Autodesk Inventor part; units mm, degrees
ref_plane "YZ Plane" through (0, 0, 0) normal (1, 0, 0) x (0, 1, 0)
ref_plane "XZ Plane" through (0, 0, 0) normal (0, 1, 0) x (-1, 0, 0)
ref_plane "XY Plane" through (0, 0, 0) normal (0, 0, 1) x (1, 0, 0)
sketch "Sketch1" plane through (0, 0, 0) normal (0, 0, 1) x (1, 0, 0)
  line L0 (0, 0) -> (236.5375, 0)
  line L1 (527.05, 0) -> (527.05, 248.2464)
  line L2 (236.5375, 266.7) -> (0, 266.7)
  line L3 (0, 266.7) -> (0, 195.5132)
  line L4 (527.05, 0) -> (101.0217, 75.1203)
  line L5 (527.05, 248.2464) -> (236.5375, 299.4716)
  line L6 (236.5375, 266.7) -> (236.5375, 299.4716)
  arc A0 (0, 195.5132) -> (101.0217, 75.1203) centre (122.2502, 195.5132) ccw
  circle A1 centre (496.8875, 187.9214) radius 3.3655
  circle A2 centre (496.8875, 60.9214) radius 3.3655
  point P0 (0, 92.9331)
  dimension "d0" = 266.7
  dimension "d2" = 10
  dimension "d3" = 244.475
  dimension "d4" = 236.5375
  dimension "d5" = 527.05
  dimension "d18" = 122.2502
  dimension "d20" = 6.731
  dimension "d21" = 60.325
  dimension "d22" = 127
  dimension "d23" = 30.1625
  dimension "d24" = 30.1625
extrude "Extrusion1" add sketch "Sketch1" along normal blind 6.35 contours L4 A0 L3 L2 L6 L5 L1 | A1 | A2
sketch "Sketch2" plane through (0, 0, 6.35) normal (0, 0, 1) x (1, 0, 0)
  line L0 (236.5375, 266.7) -> (236.5375, 299.4716)
  line L1 (0, 266.7) -> (236.5375, 266.7)
  line L2 (0, 195.5132) -> (0, 266.7)
  line L3 (527.05, 0) -> (101.0217, 75.1203)
  line L4 (527.05, 248.2464) -> (527.05, 0)
  line L5 (236.5375, 299.4716) -> (527.05, 248.2464)
  line L6 (236.5375, 294.6227) -> (527.05, 243.3976)
  line L7 (527.05, 4.8489) -> (101.8509, 79.8229)
  line L8 (4.7752, 195.5132) -> (4.7752, 266.7)
  line L9 (236.5375, 291.3988) -> (527.05, 240.1736)
  line L10 (527.05, 8.0728) -> (102.4022, 82.9497)
  line L11 (7.9502, 195.5132) -> (7.9502, 266.7)
  line L12 (4.7752, 266.7) -> (7.9502, 266.7)
  line L13 (527.05, 8.0728) -> (527.05, 4.8489)
  line L14 (236.5375, 294.6227) -> (236.5375, 291.3988)
  line L15 (527.05, 243.3976) -> (527.05, 240.1736)
  arc A0 (7.9502, 195.5132) -> (102.4022, 82.9497) centre (122.2502, 195.5132) ccw
  arc A1 (4.7752, 195.5132) -> (101.8509, 79.8229) centre (122.2502, 195.5132) ccw
  point P0 (0, 88.4544)
  point P1 (0, 0)
  point P2 (4.7752, 96.94)
  point P3 (7.9502, 99.6041)
  point P4 (101.0217, 75.1203)
  dimension "d8" = 3.175
  dimension "d9" = 4.7752
  dimension "d10" = 4.7752
  dimension "d11" = 3.175
  dimension "d12" = 4.7752
  dimension "d13" = 3.175
  dimension "d16" = 114.3
  dimension "d17" = 117.475
extrude "Extrusion2" cut sketch "Sketch2" against normal blind 3.175 contours L0 L6 L4 L9 | L11 A0 L10 L4 L7 A1 L8 L1
extrude "Extrusion3" cut sketch "Sketch1" along normal blind 25.4 contours A1 | A2
hole "Hole1" at (41.275, 254, 6.35) direction (0, 0, -1) diameter 6.35 depth 25.4 tip angle 118
pattern_linear "Rectangular Pattern1" count 3 spacing 76.2 along (1, 0, 0) of "Hole1"
equation "\"d24\" = d23"
properties part number "GE-12086-01"
Work out the finished part from the listing and answer in its coordinate system (mm). A direction names the side the tool comes from. Coordinates: 2 decimals unless noted, no trailing zeros. Loops run counter-clockwise (first coordinate to the right, second up) from the corner with the lowest first, then second, coordinate; pieces in that order, holes last. Notation, with made-up numbers: M -5,42 L 4,42 A4 ccw 4,49 Z; hole C 49,-20.5 d9. An arc over 180 degrees is marked long. Use CSV: the item, a comma, the result in double quotes. Start each with the question number.
(1) Find section D-D, the plane x = 472. Give the vertices of the cut face in (y, z) (3 decimals).
(2) Given pin 1 Ø5.5 at (x, y) = (496.89, 60.92) entering from +Z; pin 2 Ø3 at (y, z) = (279, 2.5) entering from -X; pin 3 Ø1.9 at (x, z) = (170, 3.5) entering from +Y; pin 4 Ø1 at (x, z) = (173, 4.5) entering from -Y, each flat-ended and moving along its own axis, determine where each tip first touches the part or whether it passes through.
(3) For faces 1 (the face through (383.83, 273.5, 3.13)), 2 (the face through (31.53, 120.88, 4.78)), determine the directions among +Z, -Z, +X, -X, +Y, -Y from which every point of the face is accessible in a straight line to the end or side of a thin tool.
(4) For a pull along Y with two mould halves and no side action, classify faces 3 (the face through (381, 272, 6.35)), 4 (the face through (379.76, 266.145, 4.785)), 5 (the face through (29.374, 116.021, 3.131)) as +Y half, -Y half, draft (parallel to the pull), parting line (faces both ways), or undercut.
(5) Find section A-A, the plane z = 5. State how many separate pieces and enclosed holes the cut face has, then the cut area to 3 significant figures.
(6) Find section B-B, the plane x = 229. Give the vertices of the cut face in (y, z) (3 decimals).
(7) Consider line 1 (Y direction, x = 370.5, z = 3.5); line 2 (Y direction, x = 502, z = 4); line 3 (Y direction, x = 122.5, z = 5.5). Determine where each line is inside the solid, lowest interval first.
(8) Find section C-C, the plane y = 124.5. Give the vertices of the cut face in (x, z) (3 decimals), then the cut area to 3 significant figures.
Recorded:
1,outline,"M 9.707,0 L 257.953,0 L 257.953,6.35 L 253.104,6.35 L 253.104,3.175 L 249.88,3.175 L 249.88,6.35 L 17.78,6.35 L 17.78,3.175 L 14.556,3.175 L 14.556,6.35 L 9.707,6.35 Z"
2,pin 1,"passes through"
2,pin 2,"stops at x = 236.54"
2,pin 3,"stops at y = 266.7"
2,pin 4,"stops at y = 62.34"
3,face 1,"+Z, -Z, +X, +Y"
3,face 2,"+Z"
4,face 3,"draft"
4,face 4,"undercut"
4,face 5,"-Y half"
5,separate pieces,"3"
5,enclosed holes,"5"
5,area,"113,000 mm^2"
6,outline,"M 52.554,0 L 266.7,0 L 266.7,6.35 L 60.627,6.35 L 60.627,3.175 L 57.403,3.175 L 57.403,6.35 L 52.554,6.35 Z"
7,line 1,"y = 27.6 to 32.45, 35.68 to 267.78, 271 to 275.85"
7,line 2,"y = 4.42 to 9.27, 12.49 to 244.59, 247.81 to 252.66"
7,line 3,"y = 71.33 to 76.18, 79.41 to 266.7"
8,outline,"M 22.74,0 L 527.05,0 L 527.05,6.35 L 32.687,6.35 L 32.687,3.175 L 28.669,3.175 L 28.669,6.35 L 22.74,6.35 Z"
8,area,"3,190 mm^2"
